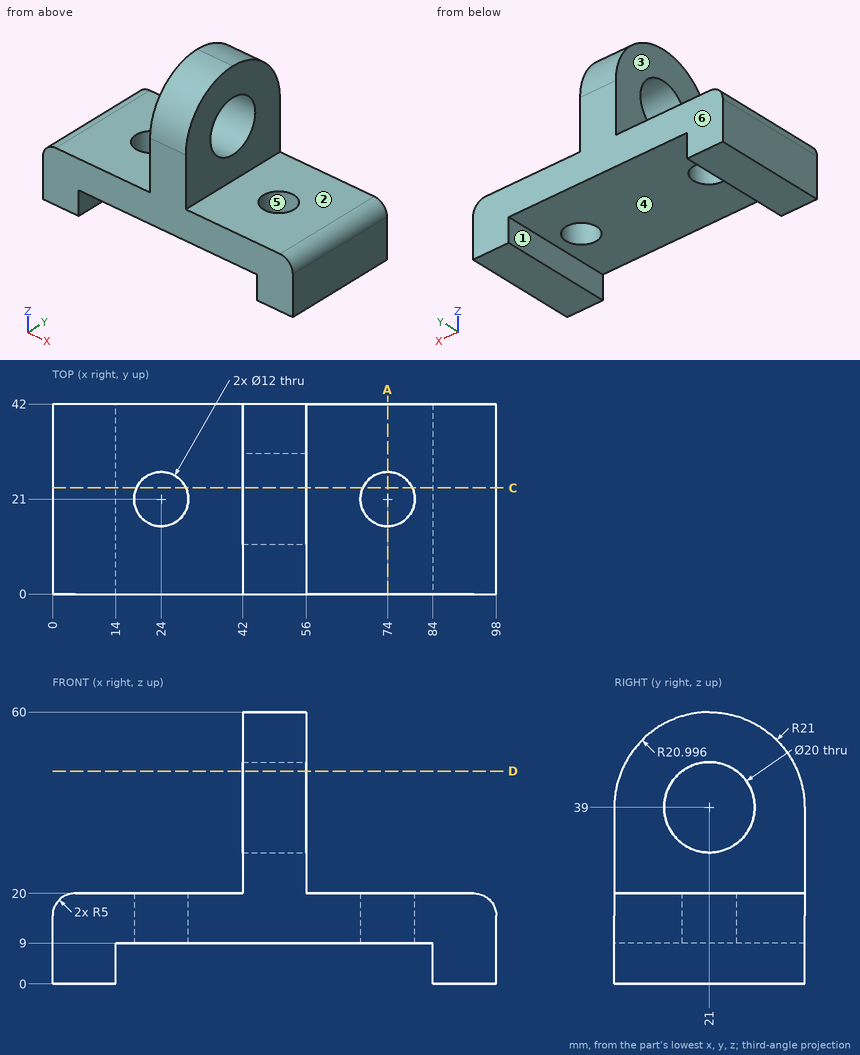
Geometry check sheet. Reference: drawing and pictorial views, mm from the part's lowest x, y, z. A direction names the side the tool comes from. Round coordinates to 2 decimals unless told otherwise and drop trailing zeros. Write each loop counter-clockwise with the first axis right and the second up, starting at its lowest first coordinate (ties: lowest second). Pieces come first, ordered by that corner, then holes.
Item 1: Go/stop test with flat-tipped pins: pin 1 Ø10 at (x, y) = (17.5, 29.5) entering from +Z; pin 2 Ø1 at (y, z) = (25, 24.5) entering from +X; pin 3 Ø12 at (y, z) = (17.5, 44) entering from -X. Record where each tip stops, or that it passes through.
Determined:
pin 1: stops at z = 20
pin 2: stops at x = 56
pin 3: stops at x = 42
Item 2: Section check D-D (z = 47). Record the boundary of the cut face in (x, y), plus the area to 3 significant figures.
Determined:
outline: (42, 1.58) - (56, 1.58) - (56, 15) - (42, 15) - close; (42, 27) - (56, 27) - (56, 40.42) - (42, 40.42) - close
area: 376 mm2
Item 3: Access from +Z, -Z, +X, -X, +Y, -Y to the whole of each face (thin tool, end or side, straight path). Record for the marked faces 1, 2 and 3.
Determined:
face 1: -Z, +Y, -Y
face 2: +Z, +X, +Y, -Y
face 3: +Z, -X, +Y, -Y
Item 4: Section check C-C (y = 23.5). Record the boundary of the cut face in (x, z).
Determined:
outline: (0, 0) - (14, 0) - (14, 9) - (18.55, 9) - (18.55, 20) - (5, 20) arc R5 ccw to (0, 15) - close; (29.45, 9) - (68.55, 9) - (68.55, 20) - (56, 20) - (56, 29.32) - (42, 29.32) - (42, 20) - (29.45, 20) - close; (42, 48.68) - (56, 48.68) - (56, 59.85) - (42, 59.85) - close; (79.45, 9) - (84, 9) - (84, 0) - (98, 0) - (98, 15) arc R5 ccw to (93, 20) - (79.45, 20) - close
Item 5: Section check A-A (x = 74). Record the boundary of the cut face in (y, z).
Determined:
outline: (0, 9) - (15, 9) - (15, 20) - (0, 20) - close; (27, 9) - (42, 9) - (42, 20) - (27, 20) - close
Item 6: Mould release check, pull along Y, two halves, no side actions. Record for the marked faces 4, 5 and 6: +Y half, -Y half, draft (parallel to the pull), parting line (faces both ways), or undercut.
Determined:
face 4: draft
face 5: undercut
face 6: +Y half
Item 7: Material ranges on line 1 along X through (y, z) = (21, 14); line 2 along X through (y, z) = (21, 16.5); line 3 along Y through (x, z) = (53, 39), recorded low to high.
Determined:
line 1: x = 0 to 18, 30 to 68, 80 to 98
line 2: x = 0.23 to 18, 30 to 68, 80 to 97.77
line 3: y = 0 to 11, 31 to 42
